from build123d import *

# Parameters (mm, degrees)
SKETCH1_W           = 80
SKETCH1_H           = 80
BOSS_EXTRUDE1_DEPTH = 25
CUT_EXTRUDE1_DEPTH  = 116.866302263


with BuildPart() as part:
    # Sketch1 → Boss-Extrude1 (new body)
    with BuildSketch(Plane(origin=(0, 0, 0), x_dir=(1, 0, 0), z_dir=(0, 1, 0))):
        with Locations((40, 40)):
            Rectangle(SKETCH1_W, SKETCH1_H)
    extrude(amount=BOSS_EXTRUDE1_DEPTH)

    # Sketch2 → Cut-Extrude1 (cut, through all)
    with BuildSketch(Plane(origin=(0, 25, 0), x_dir=(1, 0, 0), z_dir=(0, 1, 0))):
        Polygon((46.429611169, 56.894824113), (17.175992553, 72), (8, 54.229204839), (23.105175887, 46.429611169), (8, 17.175992553), (25.770795161, 8), (33.570388831, 23.105175887), (62.824007447, 8), (72, 25.770795161), (56.894824113, 33.570388831), (72, 62.824007447), (54.229204839, 72), align=None)
    extrude(amount=-CUT_EXTRUDE1_DEPTH, mode=Mode.SUBTRACT)


solid = part.part
Check sheet for the modelled part. Datum: model origin and axes. Units: mm. A direction names the side the tool comes from. Give positions to 0.01 mm unless a question says otherwise; leave off trailing zeros. Order: outer loops, then holes, each group sorted by start corner. A loop starts at its lowest first (then second) coordinate and runs counter-clockwise, first axis right, second up. Notation, with made-up numbers: M 39,2 L 92,2 A13 ccw 92,20 Z; hole C 8.5,15.25 d5. An arc over 180 degrees is marked long. Answer as CSV lines item,"result". Start each with the question number.
Item 1: Cross-section at D-D on x = 61. Enter the section's corners in (y, z).
Item 2: Mould release check, pull along Z, two halves, no side actions. Record for faces 1 (the face through (32.01, 12.68, -64.34)), 2 (the face through (29.616, 12.675, -15.447)), 3 (the face through (39, 12, -80)), 4 (the face through (13, 25, -41)): +Z half, -Z half, draft (parallel to the pull), parting line (faces both ways), or undercut.
Item 3: Cross-section at C-C on y = 6. Enter the section's corners in (x, z).
Item 4: Cross-section at B-B on z = -37. Enter the section's corners in (x, y), plus the area to 3 significant figures.
Item 5: Tool access check on faces 5 (the face through (63.239, 12.675, -67.348)), 6 (the face through (0, 12, -39)). Record the directions out of +Z, -Z, +X, -X, +Y, -Y that give a thin tool (end or side, any length) a straight path to the whole face; none if there is none.
Item 6: Cross-section at A-A on x = 49. Enter the section's corners in (y, z).
Item 7: Thickness scan on line 1 (X direction, y = 7, z = -58.5); line 2 (Z direction, x = 17.5, y = 13); line 3 (Z direction, x = 65, y = 9.5). Record the ranges inside material, lowest first. Write a range as [from, to].
Established:
1,outline,"M 0,-80 L 25,-80 L 25,-68.5 L 0,-68.5 Z; M 0,-41.52 L 25,-41.52 L 25,-31.45 L 0,-31.45 Z; M 0,-8.94 L 25,-8.94 L 25,0 L 0,0 Z"
2,face 1,"undercut"
2,face 2,"undercut"
2,face 3,"-Z half"
2,face 4,"draft"
3,outline,"M 0,-80 L 80,-80 L 80,0 L 0,0 Z; hole M 8,-54.23 L 17.18,-72 L 46.43,-56.89 L 54.23,-72 L 72,-62.82 L 56.89,-33.57 L 72,-25.77 L 62.82,-8 L 33.57,-23.11 L 25.77,-8 L 8,-17.18 L 23.11,-46.43 Z"
4,outline,"M 0,0 L 18.24,0 L 18.24,25 L 0,25 Z; M 58.67,0 L 80,0 L 80,25 L 58.67,25 Z"
4,area,"989 mm^2"
5,face 5,"+Y, -Y"
5,face 6,"+Z, -Z, -X, +Y, -Y"
6,outline,"M 0,-80 L 25,-80 L 25,-61.87 L 0,-61.87 Z; M 0,-15.14 L 25,-15.14 L 25,0 L 0,0 Z"
7,line 1,"x = [0, 10.21], [43.32, 47.26], [69.77, 80]"
7,line 2,"z = [-80, -71.83], [-49.32, -35.57], [-12.27, 0]"
7,line 3,"z = [-80, -66.44], [-49.27, -29.39], [-12.21, 0]"
